Can you work these out from the model? Positions are in its coordinate system, mm. Face numbers are marked on the shaded views. A direction names the side the tool comes from. Coordinates: 2 decimals unless noted, no trailing zeros. Order: outer loops, then holes, each group sorted by start corner. A loop starts at its lowest first (then second) coordinate and runs counter-clockwise, first axis right, second up.
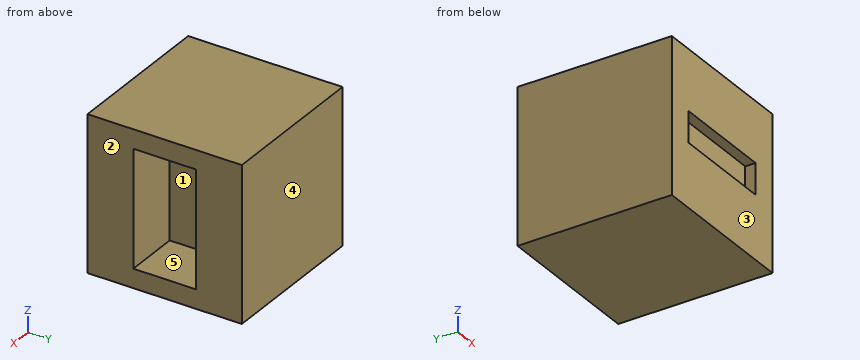
```python
from build123d import *

# Parameters (mm, degrees)
SKETCH1_W           = 30
SKETCH1_H           = 30
BOSS_EXTRUDE1_DEPTH = 30
SKETCH2_W           = 11.315
SKETCH2_H           = 6.095
CUT_EXTRUDE1_DEPTH  = 10.84
SKETCH3_W           = 20
SKETCH3_H           = 6
CUT_EXTRUDE4_DEPTH  = 2


with BuildPart() as part:
    # Sketch1 → Boss-Extrude1 (new body)
    with BuildSketch(Plane.XY):
        with Locations((15, -15)):
            Rectangle(SKETCH1_W, SKETCH1_H)
    extrude(amount=BOSS_EXTRUDE1_DEPTH)

    # Sketch2 → Cut-Extrude1 (cut)
    with BuildSketch(Plane(origin=(30, 0, 0), x_dir=(0, 0, -1), z_dir=(1, 0, 0))):
        with Locations((-20.6575, -18.0475)):
            Rectangle(SKETCH2_W, SKETCH2_H)
        Polygon((-3.685, -8.905), (-26.315, -8.905), (-26.315, -15), (-15, -15), (-3.685, -15), align=None)
        with Locations((-9.3425, -18.0475)):
            Rectangle(SKETCH2_W, SKETCH2_H)
    extrude(amount=-CUT_EXTRUDE1_DEPTH, mode=Mode.SUBTRACT)

    # Sketch3 → Cut-Extrude4 (cut)
    with BuildSketch(Plane.XZ.offset(30)):
        with Locations((14.938029793, 15.294097389)):
            Rectangle(SKETCH3_W, SKETCH3_H)
    extrude(amount=-CUT_EXTRUDE4_DEPTH, mode=Mode.SUBTRACT)


solid = part.part
```
1. Please list where these lines run through material, in increasing order: probe 1 along Y at (x, z) = (24.75, 6) (3 decimals); probe 2 along Z at (x, y) = (25.75, -10.5) (3 decimals); probe 3 along X at (y, z) = (-9.75, 12.5).
Completed:
probe 1: y = -30 to -21.095, -8.905 to 0
probe 2: z = 0 to 3.685, 26.315 to 30
probe 3: x = 0 to 19.16
2. Thinking about a two-plate mould opening in Y: for the marked faces 1, 2 and 3, which applies, pulls with the +Y half, pulls with the -Y half, needs draft (parallel to the pull), parting line crosses it, or undercut?
Completed:
face 1: undercut
face 2: needs draft
face 3: pulls with the -Y half
3. I'm going to push flat-ended pins straight in: pin 1 (3.5 mm diameter, centred on y = -15, z = 19.5, fed in from +X); pin 2 (1.8 mm diameter, centred on x = 17, z = 14.5, fed in from -Y). Where does each tip first touch, or does it pass through?
Completed:
pin 1: stops at x = 19.16
pin 2: stops at y = -28
4. Imagine slicing it at B-B on z = 7. Please give me the cut outline in (x, y) (3 decimals).
Completed:
outline: (0, -30) - (30, -30) - (30, -21.095) - (19.16, -21.095) - (19.16, -8.905) - (30, -8.905) - (30, 0) - (0, 0) - close
5. Imagine slicing it at C-C on y = -12.25. Please give me the cut outline in (x, z) (3 decimals), then the cut area to 3 significant figures.
Completed:
outline: (0, 0) - (30, 0) - (30, 3.685) - (19.16, 3.685) - (19.16, 26.315) - (30, 26.315) - (30, 30) - (0, 30) - close
area: 655 mm2
6. On a 3-axis mill with a long thin cutter (end or side, diameter ignored), from which of +Z, -Z, +X, -X, +Y, -Y can I reach the whole of each face in a straight line? I mean the marked faces 4 and 5. Say none if no direction works.
Completed:
face 4: +Z, -Z, +X, -X, +Y
face 5: +X
7. Imagine slicing it at D-D on x = 21.5. Please give me the cut outline in (y, z) (3 decimals).
Completed:
outline: (-30, 0) - (0, 0) - (0, 30) - (-30, 30) - (-30, 18.294) - (-28, 18.294) - (-28, 12.294) - (-30, 12.294) - close; hole (-21.095, 3.685) - (-8.905, 3.685) - (-8.905, 26.315) - (-21.095, 26.315) - close
8. Imagine slicing it at A-A on x = 27. Please give me the cut outline in (y, z) (3 decimals), then the cut area to 3 significant figures.
Completed:
outline: (-30, 0) - (0, 0) - (0, 30) - (-30, 30) - close; hole (-21.095, 3.685) - (-8.905, 3.685) - (-8.905, 26.315) - (-21.095, 26.315) - close
area: 624 mm2
